CAD build for the part. Positions are in the model's coordinates, mm. Face numbers are marked on the shaded views. Give positions to 0.01 mm unless a question says otherwise; leave off trailing zeros. Order: outer loops, then holes, each group sorted by start corner. A loop starts at its lowest first (then second) coordinate and runs counter-clockwise, first axis right, second up.
Autodesk Fusion 360 part; units mm, degrees
sketch "Roller_End_Cap_Outter" plane through (0, 0, 0) normal (0, 0, 1) x (1, 0, 0)
  circle A0 centre (0, 0) radius 38.1
  dimension "d2" = 76.2
extrude "Extrude1" add sketch "Roller_End_Cap_Outter" along normal blind 6.35
sketch "Roller_End_Cap_Inner" plane through (0, 0, 6.35) normal (0, 0, 1) x (-1, 0, 0)
  circle A0 centre (0, 0) radius 38.1
  circle A1 centre (0, 0) radius 34.925
  dimension "d7" = 69.85
extrude "Extrude3" add sketch "Roller_End_Cap_Inner" along normal blind 10 contours A1
sketch "Shaft Hole" plane through (0, 0, 16.35) normal (0, 0, 1) x (-1, 0, 0)
  circle A0 centre (0, 0) radius 34.925
  circle A1 centre (0, 0) radius 6.45
  dimension "d10" = 12.9
extrude "Extrude4" cut sketch "Shaft Hole" against normal through all contours A1
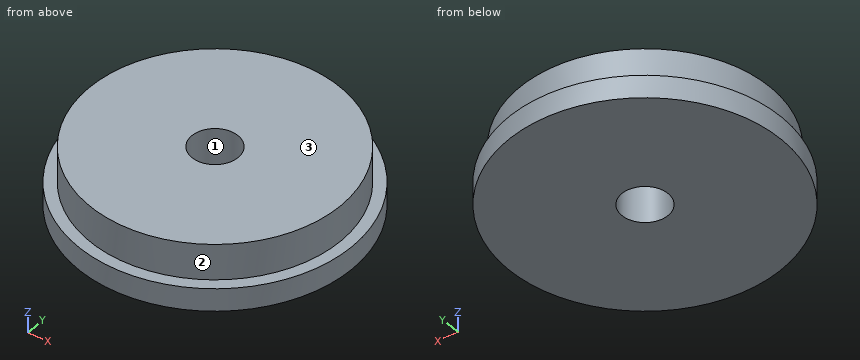
1. Saw through at A-A on x = 0. Give the cut face in (y, z) (3 decimals), plus the area to 3 significant figures.
2. Saw through at C-C on z = 10.25. Give the cut face in (x, y) (3 decimals).
3. Saw through at D-D on x = -31. Give the cut face in (y, z).
4. Mould opens along Y. For the marked faces 1, 2 and 3 say: released by +Y, released by -Y, zero draft, split by the parting line, or undercut.
5. Wall check: line 1 (Y direction, x = 0, z = 4); line 2 (Y direction, x = 0, z = 10.5) (3 decimals). Give the ranges that are in metal, low to high.
6. Pin check, flat tips, straight feed: P1, Ø6, axis at y = -14, z = 6, coming from the +X side; P2, Ø2, axis at y = 18.5, z = 9.5, coming from the +X side; P3, Ø4, axis at y = -9, z = 9, coming from the +X side. Stop position of each tip, or through.
Reported:
1. outline: (-38.1, 0) - (-6.45, 0) - (-6.45, 16.35) - (-34.925, 16.35) - (-34.925, 6.35) - (-38.1, 6.35) - close; (6.45, 0) - (38.1, 0) - (38.1, 6.35) - (34.925, 6.35) - (34.925, 16.35) - (6.45, 16.35) - close
1. area: 971 mm2
2. outline: circle Ø69.85 at (0, 0); hole circle Ø12.9 at (0, 0)
3. outline: (-22.15, 0) - (22.15, 0) - (22.15, 6.35) - (16.09, 6.35) - (16.09, 16.35) - (-16.09, 16.35) - (-16.09, 6.35) - (-22.15, 6.35) - close
4. face 1: undercut
4. face 2: split by the parting line
4. face 3: zero draft
5. line 1: y = -38.1 to -6.45, 6.45 to 38.1
5. line 2: y = -34.925 to -6.45, 6.45 to 34.925
6. P1: stops at x = 36.48
6. P2: stops at x = 30.22
6. P3: stops at x = 34.22
